```python
from build123d import *

# Parameters (mm, degrees)
SKETCH2_W               = 32.95
SKETCH2_H               = 33.638015847
BOSS_EXTRUDE1_DEPTH     = 86.1
SKETCH4_W               = 32.95
SKETCH4_H               = 14
BOSS_EXTRUDE3_DEPTH     = 33.63802
CUT_EXTRUDE1_DEPTH      = 27.1
CUT_EXTRUDE1_DEPTH_BACK = 6
CUT_EXTRUDE1_START      = -16.819008
SKETCH5_W               = 5
SKETCH5_H               = 6.8
CUT_EXTRUDE2_REACH      = 100.135
SKETCH6_W               = 5
SKETCH6_H               = 10


with BuildPart() as part:
    # Sketch2 → Boss-Extrude1 (new body)
    with BuildSketch(Plane.XY):
        with Locations((-16.475, 16.819007924)):
            Rectangle(SKETCH2_W, SKETCH2_H)
        Polygon((-5, 3.909007924), (-5, 29.729007924), (-27.95, 29.044167374), (-27.95, 4.593848474), align=None, mode=Mode.SUBTRACT)
    extrude(amount=BOSS_EXTRUDE1_DEPTH)


with BuildPart() as body_2:
    # Sketch4 → Boss-Extrude3 (new body)
    with BuildSketch(Plane(origin=(0, 0, 0), x_dir=(1, 0, 0), z_dir=(0, 1, 0))):
        with Locations((-16.475, 7)):
            Rectangle(SKETCH4_W, SKETCH4_H)
    extrude(amount=BOSS_EXTRUDE3_DEPTH)

    # Sketch5 → Cut-Extrude1 (cut, two sides: drawn at the far end of the back side and taken through both)
    with BuildSketch(Plane(origin=(0, 33.638015847, 0), x_dir=(1, 0, 0), z_dir=(0, 1, 0)).offset(CUT_EXTRUDE1_START - CUT_EXTRUDE1_DEPTH_BACK)):
        with Locations((-12, 3.4)):
            Rectangle(SKETCH5_W, SKETCH5_H)
        Polygon((-14.5, 6.8), (-9.5, 6.8), (-9.5, 7.05), (-9.5, 10.8), (-32.95, 10.8), (-32.95, 6.8), align=None)
    extrude(amount=CUT_EXTRUDE1_DEPTH + CUT_EXTRUDE1_DEPTH_BACK, mode=Mode.SUBTRACT)


with BuildPart() as part_1:
    add(part.part)

    # Combine1: union body 2
    add(body_2.part)

    # Cut-Extrude2: up to this plane
    cut_extrude2_end = Plane(origin=(-27.95, 29.044167374, 86.1), z_dir=(0.029827269826923603, -0.9995550680050959, 0))
    # Sketch6 → Cut-Extrude2 (cut, up to the surface)
    with BuildSketch(Plane(origin=(0, 33.638015847, 0), x_dir=(1, 0, 0), z_dir=(0, 1, 0)), mode=Mode.PRIVATE) as cut_extrude2_sk1:
        with Locations((-12, -5)):
            Rectangle(SKETCH6_W, SKETCH6_H)
    cut_extrude2_tool1 = split(extrude(cut_extrude2_sk1.sketch, amount=-CUT_EXTRUDE2_REACH, mode=Mode.PRIVATE), bisect_by=cut_extrude2_end, keep=Keep.BOTH, mode=Mode.PRIVATE)
    add(cut_extrude2_tool1.solids().sort_by_distance((-12, 33.638016, 5))[0], mode=Mode.SUBTRACT)


solid = part_1.part
```
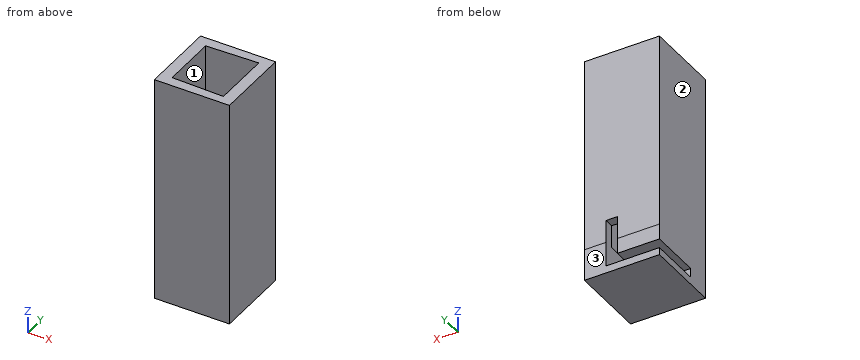
Work out the finished part from the listing and answer in its coordinate system (mm). Face numbers are marked on the shaded views. Give positions to 0.01 mm unless a question says otherwise; leave off trailing zeros. Loops run counter-clockwise (first coordinate to the right, second up) from the corner with the lowest first, then second, coordinate; pieces in that order, holes last. Notation, with made-up numbers: (2.25, -9) -> (50.25, -9) arc R9 cw to (50.25, 6) -> close; hole circle Ø3 at (16.25, -28). An arc over 180 degrees is marked (long way). Write item = value, one per line. Start each with the question number.
(1) Find section A-A on z = 69. Give the vertices of the cut face in (x, y), and give its area (3 significant figures).
(2) Find section B-B on y = 17. Give the vertices of the cut face in (x, z), and give its area (3 significant figures).
(3) Find section D-D on x = -13. Give the vertices of the cut face in (y, z).
(4) Find the intervals of material crossed by probe 1 along X at (y, z) = (29, 76); probe 2 along Z at (x, y) = (-27, 24); probe 3 along Z at (x, y) = (-13, 10.5), in increasing order. Write a range as from..to.
(5) The mould has two halves that part along X. Classify the marked faces 1, 2 and 3: +X half, -X half, draft (parallel to the pull), parting line (faces both ways), or undercut.
(6) Given pin 1 Ø5 at (y, z) = (14, 3) entering from +X; pin 2 Ø11.5 at (x, y) = (-17.5, 22.5) entering from +Z, each flat-ended and moving along its own axis, determine where each tip first touches the part or whether it passes through.
From the geometry:
q1.outline = (-32.95, 0) -> (0, 0) -> (0, 33.64) -> (-32.95, 33.64) -> close; hole (-27.95, 4.59) -> (-5, 3.91) -> (-5, 29.73) -> (-27.95, 29.04) -> close
q1.area = 532 mm^2
q2.outline = (-32.95, -14) -> (0, -14) -> (0, 86.1) -> (-5, 86.1) -> (-5, 0) -> (-9.5, 0) -> (-9.5, -10.8) -> (-32.95, -10.8) -> close; (-32.95, -6.8) -> (-14.5, -6.8) -> (-14.5, 0) -> (-27.95, 0) -> (-27.95, 86.1) -> (-32.95, 86.1) -> close
q2.area = 1,190 mm^2
q3.outline = (0, -14) -> (33.64, -14) -> (33.64, -10.8) -> (10.82, -10.8) -> (10.82, 0) -> (4.15, 0) -> (4.15, 86.1) -> (0, 86.1) -> close; (29.49, 10) -> (33.64, 10) -> (33.64, 86.1) -> (29.49, 86.1) -> close
q4.probe_1 = -32.95..-27.95, -5..0
q4.probe_2 = -14..-10.8, -6.8..0
q4.probe_3 = -14..0
q5.face_1 = undercut
q5.face_2 = -X half
q5.face_3 = draft
q6.pin_1 = 0
q6.pin_2 = 0
